Source: CAD feature listing. Evaluate the final solid. Frame: model axes, mm. Face numbers are marked on the shaded views. A direction names the side the tool comes from. Round coordinates to 2 decimals unless told otherwise and drop trailing zeros. Write each loop counter-clockwise with the first axis right and the second up, starting at its lowest first coordinate (ties: lowest second). Pieces come first, ordered by that corner, then holes. Notation, with made-up numbers: M 14,20 L 30,20 A13 ccw 30,25 Z; hole C 48.25,44 d11. An arc over 180 degrees is marked long. Use a Markdown table: item, result.
```python
from build123d import *

# Parameters (mm, degrees)
F0_W        = 60
F0_H        = 60
F1_DEPTH    = 25
F2_W        = 50
F2_H        = 50
F3_DEPTH    = 25
F4_R        = 5
F5_R        = 2
F6_DEPTH    = 28
F7_R        = 3.5
F8_DEPTH    = 5
F9_S5_R     = 3.5
F9_T6_DEPTH = 12
F10_SIZE    = 4


# Not quite as in the source:
# - a fillet or chamfer that OpenCascade refuses, or shapes differently, is made with other operations: its cross-section is extruded or revolved along the edge and cut away or added


with BuildPart() as f1:
    # F0 (on Top) → F1 (new body)
    with BuildSketch(Plane.XY):
        with Locations((3.075433895, 2.043666031)):
            Rectangle(F0_W, F0_H)
    extrude(amount=F1_DEPTH)

    # F2 (on face) → F3 (cut)
    with BuildSketch(Plane.XY.offset(25)):
        with Locations((8.075433895, 7.043666031)):
            Rectangle(F2_W, F2_H)
    extrude(amount=-F3_DEPTH, mode=Mode.SUBTRACT)

    # F4
    f4_edges = [f1.edges().sort_by_distance(p)[0] for p in [
        (-26.924566, -27.956334, 12.5),
    ]]
    fillet(f4_edges, radius=F4_R)

    # F5 (on face) → F6 (cut)
    with BuildSketch(Plane.XY.offset(25)):
        with Locations((-21.924566105, 24.043666031)):
            Circle(F5_R)
        with Locations((-21.924566105, -22.1858429265)):
            Circle(F5_R)
        with Locations((25.075433895, -22.956333969)):
            Circle(F5_R)
    extrude(amount=-F6_DEPTH, mode=Mode.SUBTRACT)

    # F7 (on face) → F8 (cut)
    with BuildSketch(Plane.XY.offset(25)):
        with Locations((-21.924566105, 24.043666031)):
            Circle(F7_R)
        with Locations((25.075433895, -22.956333969)):
            Circle(F7_R)
        with Locations((-21.924566105, -22.1858429265)):
            Circle(F7_R)
    extrude(amount=-F8_DEPTH, mode=Mode.SUBTRACT)

    # F9: chamfer of 5 on 1 edges, made by hand


with BuildPart() as f9_tool2:
    # F9_s3 → F9_t4 (revolve)
    with BuildSketch(Plane.XZ.offset(22.1858429265)):
        Polygon((-19.924566105, 15), (-14.924566105, 20), (-19.924566105, 20), align=None)
    revolve(axis=Axis((-21.924566105, -22.1858429265, 20), (0, 0, 1)))

    # F9_s5 → F9_t6 (intersect, symmetric)
    with BuildSketch(Plane.XY.offset(17.5)):
        with Locations((-21.924566105, -22.1858429265)):
            Circle(F9_S5_R)
    extrude(amount=F9_T6_DEPTH, both=True, mode=Mode.INTERSECT)


with BuildPart() as f1_1:
    add(f1.part)

    # F9_t1: cut F9_tool2
    add(f9_tool2.part, mode=Mode.SUBTRACT)

    # F10
    f10_edges = [f1_1.edges().sort_by_distance(p)[0] for p in [
        (-26.924566, 32.043666, 12.5),
        (33.075434, -27.956334, 12.5),
    ]]
    chamfer(f10_edges, length=F10_SIZE)


solid = f1_1.part
```
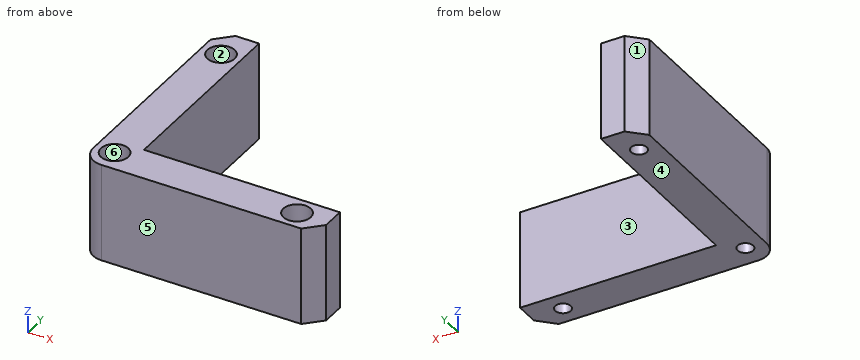
Q1. Reachability of the marked faces 1, 2 and 3 from +Z, -Z, +X, -X, +Y, -Y: full face, straight path, thin tool, end or side. Return the list, or none.
Results are:
| item | result |
|---|---|
| face 1 | +Z, -Z, -X, +Y |
| face 2 | +Z |
| face 3 | +Z, -Z, +X, +Y |
Q2. Section D-D on z = 21.75. Return loops of the section in (x, y), plus the area to 3 significant figures.
Results are:
| item | result |
|---|---|
| outline | M -26.92,-22.96 A5 ccw -21.92,-27.96 L 29.08,-27.96 L 33.08,-23.96 L 33.08,-17.96 L -16.92,-17.96 L -16.92,32.04 L -22.92,32.04 L -26.92,28.04 Z; hole C -21.92,-22.19 d7; hole C -21.92,24.04 d7; hole C 25.08,-22.96 d7 |
| area | 963 mm^2 |
Q3. Line query: L1, parallel to Y at x = 15, z = 12.75; L2, parallel to X at y = -16, z = 6; L3, parallel to X at y = -23.5, z = 2. Output: solid intervals per line, ascending.
Results are:
| item | result |
|---|---|
| L1 | -27.96 to -17.96 |
| L2 | -26.92 to -16.92 |
| L3 | -26.89 to -23.43, -20.42 to 23.15, 27 to 33.08 |
Q4. First-contact query: pin 1 Ø3.5 at (x, y) = (25, -23) entering from +Z; pin 2 Ø6.5 at (x, y) = (-21.92, 24.04) entering from +Z; pin 3 Ø12.5 at (y, z) = (-0.5, 8.5) entering from +X; pin 4 Ø5 at (x, y) = (-21.92, -22.19) entering from +Z. Flat tips, straight axial feed; report the tip coordinate or a pass-through.
Results are:
| item | result |
|---|---|
| pin 1 | through |
| pin 2 | z = 20 |
| pin 3 | x = -16.92 |
| pin 4 | z = 15.51 |
Q5. Section A-A on z = 9. Return loops of the section in (x, y).
Results are:
| item | result |
|---|---|
| outline | M -26.92,-22.96 A5 ccw -21.92,-27.96 L 29.08,-27.96 L 33.08,-23.96 L 33.08,-17.96 L -16.92,-17.96 L -16.92,32.04 L -22.92,32.04 L -26.92,28.04 Z; hole C -21.92,-22.19 d4; hole C -21.92,24.04 d4; hole C 25.08,-22.96 d4 |
Q6. Section C-C on y = 3.5. Return loops of the section in (x, z), plus the area to 3 significant figures.
Results are:
| item | result |
|---|---|
| outline | M -26.92,0 L -16.92,0 L -16.92,25 L -26.92,25 Z |
| area | 250 mm^2 |
Q7. Mould query, pull axis Y, two halves, no side actions, for the marked faces 4, 5 and 6. Classes: +Y half, -Y half, draft (parallel to the pull), parting line (faces both ways), or undercut.
Results are:
| item | result |
|---|---|
| face 4 | draft |
| face 5 | -Y half |
| face 6 | undercut |
Q8. Section B-B on x = 16. Return loops of the section in (y, z).
Results are:
| item | result |
|---|---|
| outline | M -27.96,0 L -17.96,0 L -17.96,25 L -27.96,25 Z |
